Source: three-view drawing plus pictorial views. Frame: mm from the lowest corner of the part. A direction names the side the tool comes from. Give positions to 0.01 mm unless a question says otherwise; leave off trailing zeros. Write each loop counter-clockwise with the first axis right and the second up, starting at its lowest first coordinate (ties: lowest second). Pieces come first, ordered by that corner, then holes. Notation, with made-up numbers: M 64.25,-22 L 104.25,-22 A28 ccw 104.25,3 Z; hole C -32,-14.75 d3. An arc over 180 degrees is marked long. Return JSON: item names as keys, results as strings.
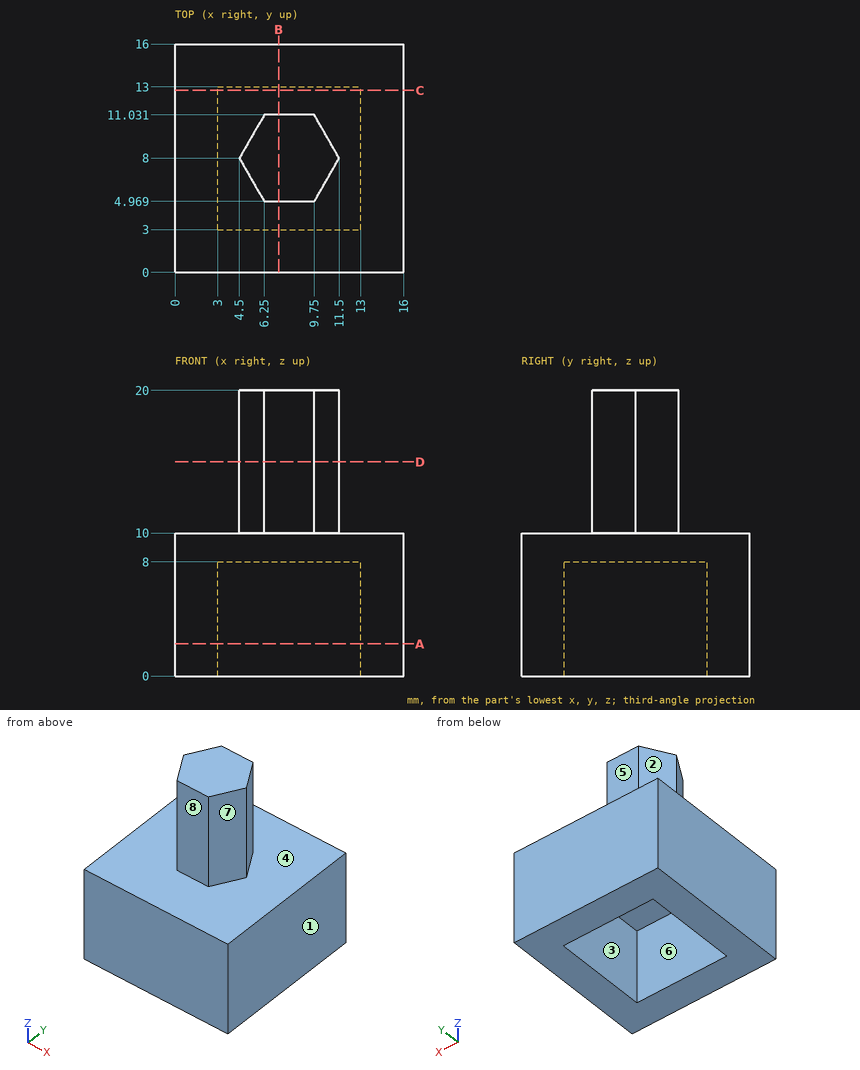
1) Cut plane A-A, the plane z = 2.25. Return the cut outline in (x, y), then the cut area to 3 significant figures.
Numbers:
{"outline": "M 0,0 L 16,0 L 16,16 L 0,16 Z; hole M 3,3 L 13,3 L 13,13 L 3,13 Z", "area": "156 mm²"}
2) Draft query along X for the marked faces 6, 7 and 8. Return one class per face: released by +X, released by -X, zero draft, split by the parting line, or undercut.
Numbers:
{"face 6": "undercut", "face 7": "released by +X", "face 8": "zero draft"}
3) Cut plane C-C, the plane y = 12.75. Return the cut outline in (x, z), then the cut area to 3 significant figures.
Numbers:
{"outline": "M 0,0 L 3,0 L 3,8 L 13,8 L 13,0 L 16,0 L 16,10 L 0,10 Z", "area": "80.0 mm²"}
4) Cut plane D-D, the plane z = 15. Return the cut outline in (x, y), then the cut area to 3 significant figures.
Numbers:
{"outline": "M 4.5,8 L 6.25,4.97 L 9.75,4.97 L 11.5,8 L 9.75,11.03 L 6.25,11.03 Z", "area": "31.8 mm²"}
5) Set-up query: the marked faces 1, 2, 3, 4 and 5. Return all of +Z, -Z, +X, -X, +Y, -Y with unobstructed straight access to the full face (end or side cutting, diameter ignored); none if empty.
Numbers:
{"face 1": "+Z, -Z, +X, +Y, -Y", "face 2": "+Z, -X, +Y", "face 3": "-Z", "face 4": "+Z", "face 5": "+Z, +X, -X, +Y"}
6) Contact query for flat-ended pins moving along their axis: pin 1 Ø1.5 at (y, z) = (4.5, 17) entering from +X; pin 2 Ø4 at (x, z) = (8, 14) entering from +Y; pin 3 Ø1 at (y, z) = (12, 13) entering from -X; pin 4 Ø6 at (y, z) = (11.5, 16) entering from +X. Output: stop coordinate, or through.
Numbers:
{"pin 1": "stops at x = 9.91", "pin 2": "stops at y = 11.03", "pin 3": "passes through", "pin 4": "stops at x = 11.21"}
7) Cut plane B-B, the plane x = 7.25. Return the cut outline in (y, z), then the cut area to 3 significant figures.
Numbers:
{"outline": "M 0,0 L 3,0 L 3,8 L 13,8 L 13,0 L 16,0 L 16,10 L 11.03,10 L 11.03,20 L 4.97,20 L 4.97,10 L 0,10 Z", "area": "141 mm²"}
8) Line query: line 1 (Y direction, x = 8, z = 3.75); line 2 (Z direction, x = 6.75, y = 5.75). Output: solid intervals per line, ascending. Write a range as [from, to].
Numbers:
{"line 1": "y = [0, 3], [13, 16]", "line 2": "z = [8, 20]"}
